Study the drawing (mm; zero at the part's minimum x, y, z) and answer. A direction names the side the tool comes from. Coordinates: 2 decimals unless noted, no trailing zeros. Write each loop counter-clockwise with the first axis right and the second up, starting at its lowest first coordinate (ties: lowest second). Pieces come first, ordered by that corner, then holes. Notation, with made-up numbers: (63, 60) -> (83, 60) arc R23 ccw to (83, 74) -> close; hole circle Ø2 at (32.25, -9). An arc over 180 degrees is marked (long way). Write item = value, one per line. Start each with the question number.
1) Flat-ended cylindrical pins translate along their axes: pin 1 Ø1.5 at (x, y) = (17.5, 38) entering from +Z (1 decimal); pin 2 Ø1 at (x, z) = (4, 9.5) entering from +Y; pin 3 Ø3 at (x, y) = (17, 39.5) entering from +Z; pin 4 Ø6 at (x, y) = (3, 37) entering from +Z. Find the tip coordinate at first contact, or state that the pin passes through.
2) A tool of negligible diameter and unlimited length cuts with its end or side. For the marked faces 1 and 2, from which of +Z, -Z, +X, -X, +Y, -Y can it reach the whole face along a straight path? Write none if from no direction.
3) Section B-B (x = 12.7) is taken. Determine the outline of the cut face in (y, z).
4) For a pull along Z with two mould halves and no side action, classify the marked faces 3, 4, 5 and 6 as released by +Z, released by -Z, zero draft, split by the parting line, or undercut.
5) Section C-C (y = 28.5) is taken. Determine the outline of the cut face in (x, z) (1 decimal).
6) Section A-A (z = 25.4) is taken. Determine the outline of the cut face in (x, y).
7) Section D-D (x = 20.75) is taken. Determine the outline of the cut face in (y, z), plus the area to 3 significant figures.
8) Find the intervals of material crossed by line 1 along Z through (x, y) = (12.75, 41) (1 decimal); line 2 along Y through (x, z) = (1.75, 28.5); line 3 along X through (y, z) = (31.5, 16), in increasing order. Write a range as from..to.
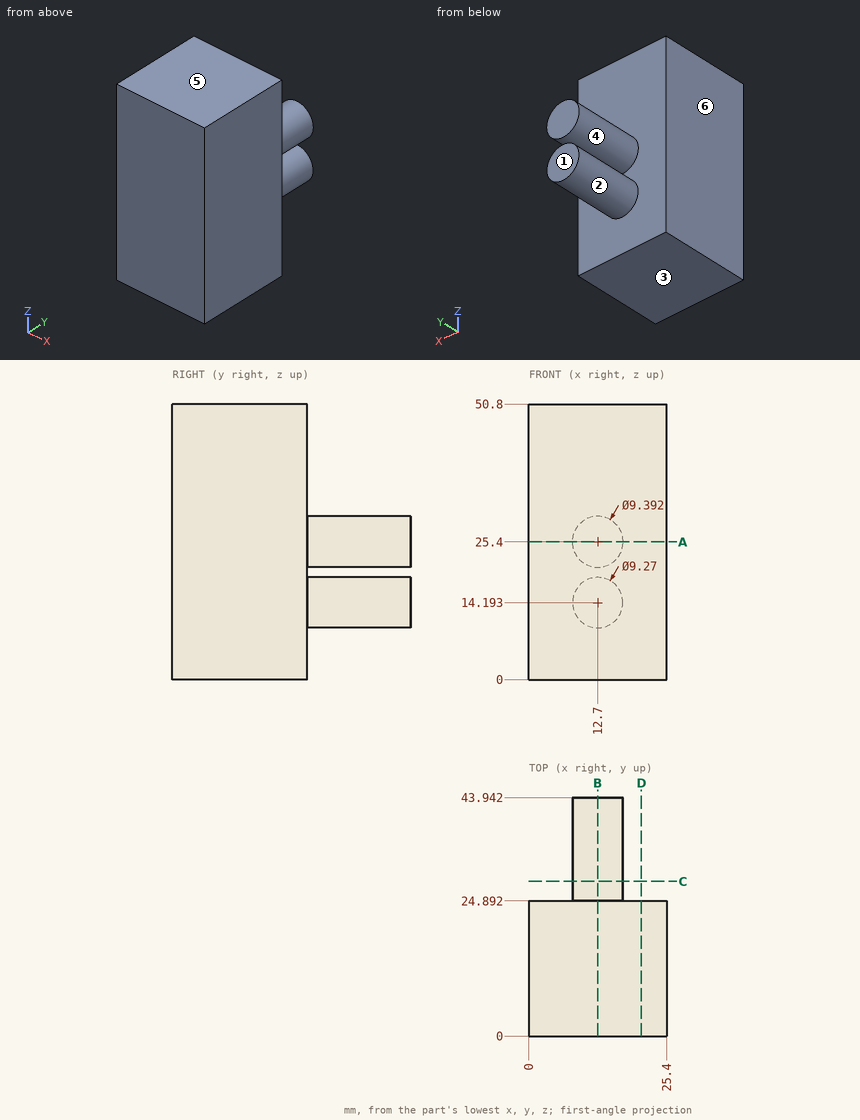
Answer key:
q1.pin_1 = 27.8
q1.pin_2 = 24.89
q1.pin_3 = 29.17
q1.pin_4 = through
q2.face_1 = +Z, -Z, +X, -X, +Y
q2.face_2 = +Y
q3.outline = (0, 0) -> (24.89, 0) -> (24.89, 9.56) -> (43.94, 9.56) -> (43.94, 18.83) -> (24.89, 18.83) -> (24.89, 20.7) -> (43.94, 20.7) -> (43.94, 30.1) -> (24.89, 30.1) -> (24.89, 50.8) -> (0, 50.8) -> close
q4.face_3 = released by -Z
q4.face_4 = undercut
q4.face_5 = released by +Z
q4.face_6 = zero draft
q5.outline = circle Ø9.4 at (12.7, 25.4); circle Ø9.3 at (12.7, 14.2)
q6.outline = (0, 0) -> (25.4, 0) -> (25.4, 24.89) -> (17.4, 24.89) -> (17.4, 43.94) -> (8, 43.94) -> (8, 24.89) -> (0, 24.89) -> close
q7.outline = (0, 0) -> (24.89, 0) -> (24.89, 50.8) -> (0, 50.8) -> close
q7.area = 1,260 mm^2
q8.line_1 = 9.6..18.8, 20.7..30.1
q8.line_2 = 0..24.89
q8.line_3 = 8.43..16.97
